For this review, use the dimensioned drawing (mm, ordinates from the lowest corner) and the shaded views. Give positions to 0.01 mm unless a question says otherwise; leave off trailing zeros. Order: outer loops, then holes, each group sorted by start corner. A loop starts at its lowest first (then second) coordinate and runs counter-clockwise, first axis right, second up. Notation, with made-up numbers: (-30, -35.5) - (1, -35.5) arc R14 cw to (1, -18.5) - close; hole circle Ø8 at (41, 30.5). An arc over 180 degrees is marked (long way). Use a Markdown table: item, result. Add a question column.
1) We need section A-A on y = 109.5. Write out the cut boundary in (x, z), then the cut area to 3 significant figures.
2) We need section C-C on z = 28. Write out the cut boundary in (x, y).
3) Wall thickness on L1, parallel to Y at x = 109, z = 13; L2, parallel to X at y = 142, z = 23.5: over which ranges is each line inside the solid? List them lowest first.
4) We need section D-D on y = 39. Write out the cut boundary in (x, z), then the cut area to 3 significant figures.
5) Mouldability with a two-part tool opening along X and no side actions: class the marked faces 1, 2 and 3 as released by +X, released by -X, zero draft, split by the parting line, or undercut.
6) Clearance check with flat-ended pins moving along their axes: P1, Ø8, axis at y = 172.5, z = 10.5, coming from the +X side; P2, Ø5, axis at y = 34.5, z = 33.5, coming from the -X side; P3, Ø4, axis at y = 114.5, z = 29, coming from the -X side. State where each tip first meets the part, or that it passes through.
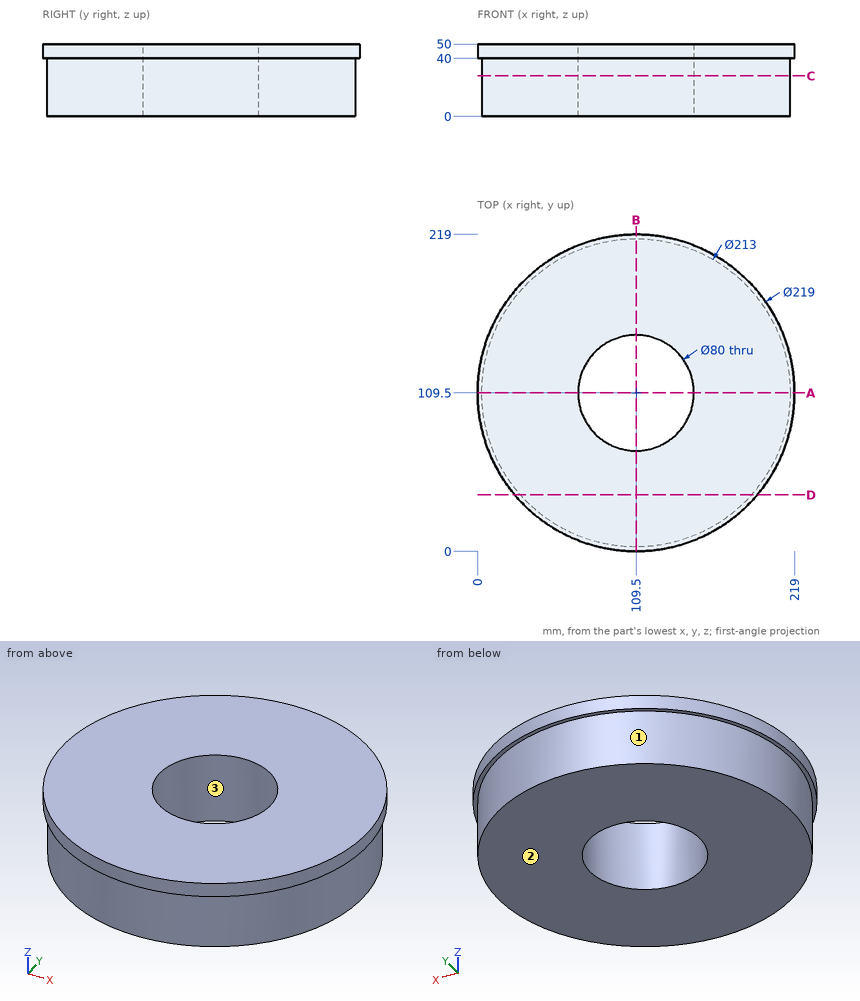
Checked values:
| question | item | result |
|---|---|---|
| 1 | outline | (0, 40) - (3, 40) - (3, 0) - (69.5, 0) - (69.5, 50) - (0, 50) - close; (149.5, 0) - (216, 0) - (216, 40) - (219, 40) - (219, 50) - (149.5, 50) - close |
| 1 | area | 6,710 mm² |
| 2 | outline | circle Ø213 at (109.5, 109.5); hole circle Ø80 at (109.5, 109.5) |
| 3 | L1 | 3 to 69.5, 149.5 to 216 |
| 3 | L2 | 8.08 to 86.18, 132.82 to 210.92 |
| 4 | outline | (25.71, 40) - (29.68, 40) - (29.68, 0) - (189.32, 0) - (189.32, 40) - (193.29, 40) - (193.29, 50) - (25.71, 50) - close |
| 4 | area | 8,060 mm² |
| 5 | face 1 | split by the parting line |
| 5 | face 2 | zero draft |
| 5 | face 3 | undercut |
| 6 | P1 | x = 198.16 |
| 6 | P2 | x = 31.49 |
| 6 | P3 | x = 3.04 |
